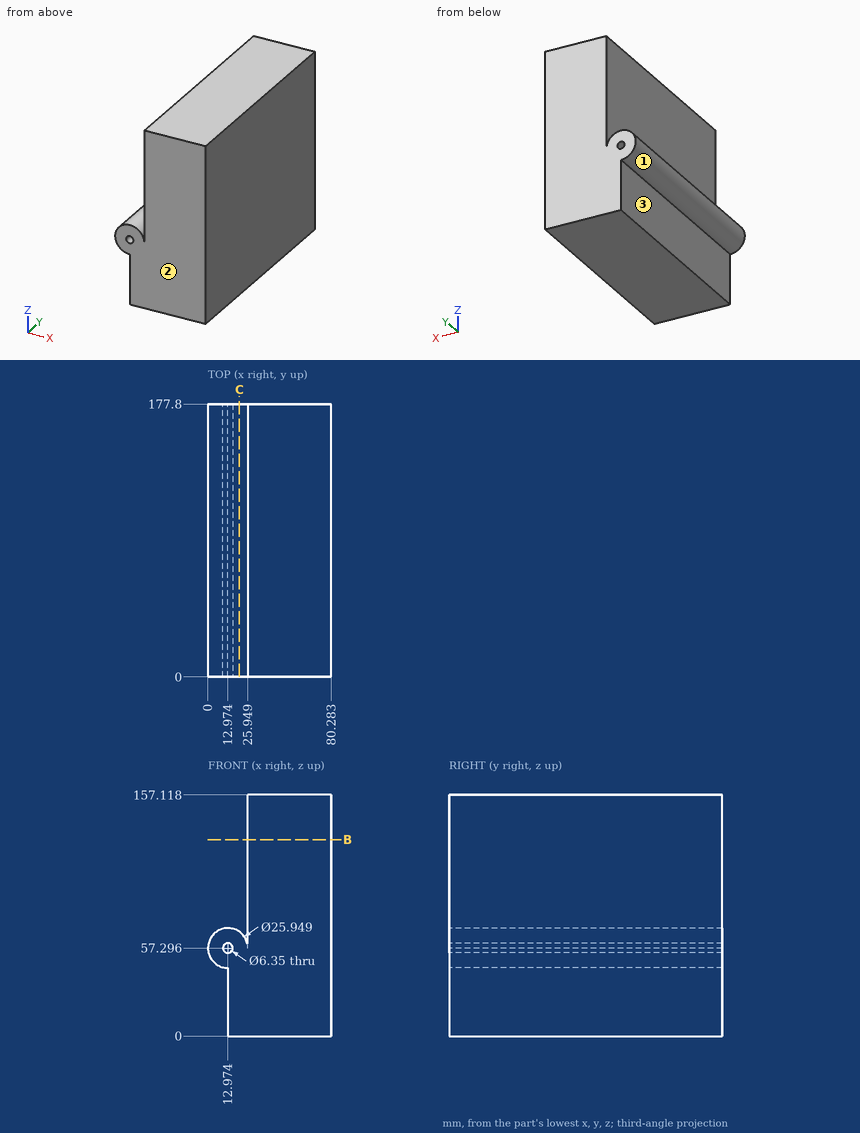
Here's the drawing with two shaded views (mm, measured from the low corner). I have some questions. Round coordinates to 2 decimals unless told otherwise and drop trailing zeros. Loops run counter-clockwise (first coordinate to the right, second up) from the corner with the lowest first, then second, coordinate; pieces in that order, holes last. Notation, with made-up numbers: (85, -19.5) - (128, -19.5) arc R14 ccw to (128, -12.5) - close; hole circle Ø2 at (1, 71). An arc over 180 degrees is marked (long way). Use CSV: the item, a comma, the result in double quotes. Start each with the question number.
1) We'd pull the mould along X, two halves only. Please class the marked faces 1, 2 and 3: released by +X, released by -X, zero draft, split by the parting line, or undercut.
2) Please list where these lines run through material, in increasing order: probe 1 along X at (y, z) = (158.5, 83.5); probe 2 along X at (y, z) = (137.5, 18) (1 decimal); probe 3 along Z at (x, y) = (12, 71.5) (1 decimal). Write a range as [from, to].
3) For pin 1 Ø8 at (x, y) = (8.5, 117) entering from -Z; pin 2 Ø22 at (y, z) = (90, 19.5) entering from -X, each with a flat end and sliding along its axis, tell me the tip position at first contact or that it passes through.
4) If we section it at C-C on x = 20.5: Write out the boundary of the cut face in (y, z) (1 decimal), plus the area to 3 significant figures.
5) If we section it at B-B on z = 128: Write out the boundary of the cut face in (x, y), plus the area to 3 significant figures.
Geometry results:
1,face 1,"undercut"
1,face 2,"zero draft"
1,face 3,"released by -X"
2,probe 1,"x = [25.95, 80.28]"
2,probe 2,"x = [13, 80.3]"
2,probe 3,"z = [44.4, 54.3], [60.3, 70.2]"
3,pin 1,"stops at z = 44.33"
3,pin 2,"stops at x = 12.97"
4,outline,"(0, 0) - (177.8, 0) - (177.8, 67.9) - (0, 67.9) - close"
4,area,"12,100 mm2"
5,outline,"(25.95, 0) - (80.28, 0) - (80.28, 177.8) - (25.95, 177.8) - close"
5,area,"9,660 mm2"
